```python
from build123d import *

# Parameters (mm, degrees)
F1_DEPTH = 25.4
F2_DEPTH = 50.8


with BuildPart() as f1:
    # F0 (on Top) → F1 (new body)
    with BuildSketch(Plane.XY):
        with BuildLine():
            Line((-22.589232, -50.8), (0, -50.8))
            Line((0, -50.8), (22.589232, -50.8))
            ThreePointArc((22.589232, -50.8), (29.879351, -49.349905), (36.059616, -45.220384))
            Line((36.059616, -45.220384), (45.220384, -36.059616))
            ThreePointArc((45.220384, -36.059616), (49.349905, -29.879351), (50.8, -22.589232))
            Line((50.8, -22.589232), (50.8, 0))
            Line((50.8, 0), (50.8, 22.589232))
            ThreePointArc((50.8, 22.589232), (49.349905, 29.879351), (45.220384, 36.059616))
            Line((45.220384, 36.059616), (36.059616, 45.220384))
            ThreePointArc((36.059616, 45.220384), (29.879351, 49.349905), (22.589232, 50.8))
            Line((22.589232, 50.8), (0, 50.8))
            Line((0, 50.8), (-22.589232, 50.8))
            ThreePointArc((-22.589232, 50.8), (-29.879351, 49.349905), (-36.059616, 45.220384))
            Line((-36.059616, 45.220384), (-45.220384, 36.059616))
            ThreePointArc((-45.220384, 36.059616), (-49.349905, 29.879351), (-50.8, 22.589232))
            Line((-50.8, 22.589232), (-50.8, 0))
            Line((-50.8, 0), (-50.8, -22.589232))
            ThreePointArc((-50.8, -22.589232), (-49.349905, -29.879351), (-45.220384, -36.059616))
            Line((-45.220384, -36.059616), (-36.059616, -45.220384))
            ThreePointArc((-36.059616, -45.220384), (-29.879351, -49.349905), (-22.589232, -50.8))
        make_face()
    extrude(amount=F1_DEPTH)

    # F0 (on Top) → F2 (join)
    with BuildSketch(Plane.XY):
        with BuildLine():
            ThreePointArc((54.20064, -45.039872), (61.083175, -34.739431), (63.5, -22.589232))
            Line((63.5, -22.589232), (63.5, 0))
            Line((63.5, 0), (63.5, 22.589232))
            ThreePointArc((63.5, 22.589232), (61.083175, 34.739431), (54.20064, 45.039872))
            Line((54.20064, 45.039872), (45.039872, 54.20064))
            ThreePointArc((45.039872, 54.20064), (34.739431, 61.083175), (22.589232, 63.5))
            Line((22.589232, 63.5), (0, 63.5))
            Line((0, 63.5), (-22.589232, 63.5))
            ThreePointArc((-22.589232, 63.5), (-34.739431, 61.083175), (-45.039872, 54.20064))
            Line((-45.039872, 54.20064), (-54.20064, 45.039872))
            ThreePointArc((-54.20064, 45.039872), (-61.083175, 34.739431), (-63.5, 22.589232))
            Line((-63.5, 22.589232), (-63.5, 0))
            Line((-63.5, 0), (-63.5, -22.589232))
            ThreePointArc((-63.5, -22.589232), (-61.083175, -34.739431), (-54.20064, -45.039872))
            Line((-54.20064, -45.039872), (-45.039872, -54.20064))
            ThreePointArc((-45.039872, -54.20064), (-34.739431, -61.083175), (-22.589232, -63.5))
            Line((-22.589232, -63.5), (0, -63.5))
            Line((0, -63.5), (22.589232, -63.5))
            ThreePointArc((22.589232, -63.5), (34.739431, -61.083175), (45.039872, -54.20064))
            Line((45.039872, -54.20064), (54.20064, -45.039872))
        make_face()
        with BuildLine():
            Line((22.589232, -50.8), (0, -50.8))
            Line((0, -50.8), (-22.589232, -50.8))
            ThreePointArc((-22.589232, -50.8), (-29.879351, -49.349905), (-36.059616, -45.220384))
            Line((-36.059616, -45.220384), (-45.220384, -36.059616))
            ThreePointArc((-45.220384, -36.059616), (-49.349905, -29.879351), (-50.8, -22.589232))
            Line((-50.8, -22.589232), (-50.8, 0))
            Line((-50.8, 0), (-50.8, 22.589232))
            ThreePointArc((-50.8, 22.589232), (-49.349905, 29.879351), (-45.220384, 36.059616))
            Line((-45.220384, 36.059616), (-36.059616, 45.220384))
            ThreePointArc((-36.059616, 45.220384), (-29.879351, 49.349905), (-22.589232, 50.8))
            Line((-22.589232, 50.8), (0, 50.8))
            Line((0, 50.8), (22.589232, 50.8))
            ThreePointArc((22.589232, 50.8), (29.879351, 49.349905), (36.059616, 45.220384))
            Line((36.059616, 45.220384), (45.220384, 36.059616))
            ThreePointArc((45.220384, 36.059616), (49.349905, 29.879351), (50.8, 22.589232))
            Line((50.8, 22.589232), (50.8, 0))
            Line((50.8, 0), (50.8, -22.589232))
            ThreePointArc((50.8, -22.589232), (49.349905, -29.879351), (45.220384, -36.059616))
            Line((45.220384, -36.059616), (36.059616, -45.220384))
            ThreePointArc((36.059616, -45.220384), (29.879351, -49.349905), (22.589232, -50.8))
        make_face(mode=Mode.SUBTRACT)
    extrude(amount=F2_DEPTH)


solid = f1.part
```
The listing builds one solid part. Answer for the finished solid, in the listing's coordinates (mm). A direction names the side the tool comes from. Coordinates: 2 decimals unless noted, no trailing zeros. Write each loop counter-clockwise with the first axis right and the second up, starting at its lowest first coordinate (ties: lowest second). Pieces come first, ordered by that corner, then holes. Notation, with made-up numbers: (56, 31.5) - (100, 31.5) arc R20 cw to (100, 59.5) - close; hole circle Ø6 at (-38.5, 36.25). An arc over 180 degrees is marked (long way). Return JSON: item names as keys, results as strings. Group by question number.
Q1. For a pull along X with two mould halves and no side action, classify faces 1 (the cylindrical face through (-61.016, 34.901, 25.044)), 2 (the cylindrical face through (-49.39, 29.78, 37.92)), 3 (the flat face through (-1, 1, 0)) as +X half, -X half, draft (parallel to the pull), parting line (faces both ways), or undercut.
Q2. Flat-ended cylindrical pins translate along their axes: pin 1 Ø5 at (x, z) = (-42, 15) entering from -Y; pin 2 Ø5 at (x, y) = (37, -5.5) entering from -Z; pin 3 Ø6 at (x, y) = (-28.5, -2.5) entering from +Z; pin 4 Ø6 at (y, z) = (28.5, 45.5) entering from -X. Find the tip coordinate at first contact, or state that the pin passes through.
Q3. Which of the six approach directions +Z, -Z, +X, -X, +Y, -Y give full straight-line access (tool end or side, diameter ignored) to faces 4 (the cylindrical face through (34.901, 61.016, 25.044)), 5 (the flat face through (50.8, 0, 38))?
Q4. Find the intervals of material crossed by line 1 along X through (y, z) = (-20.5, 31.5); line 2 along Z through (x, y) = (31, 36), in increasing order. Write a range as [from, to].
Q5. The part is cut by section D-D on z = 22.5. Write down the section's boundary in (x, y), and give its area (3 significant figures).
Q6. The part is cut by section A-A on x = -10. Write down the section's boundary in (y, z).
Evaluation:
{
 "1": {"face 1": "-X half", "face 2": "undercut", "face 3": "draft"},
 "2": {"pin 1": "stops at y = -58.62", "pin 2": "stops at z = 0", "pin 3": "stops at z = 25.4", "pin 4": "stops at x = -63.37"},
 "3": {"face 4": "+Z, -Z, +X, +Y", "face 5": "+Z"},
 "4": {"line 1": "x = [-63.5, -50.8], [50.8, 63.5]", "line 2": "z = [0, 25.4]"},
 "5": {"outline": "(-63.5, -22.59) arc R31.75 ccw to (-54.2, -45.04) - (-45.04, -54.2) arc R31.75 ccw to (-22.59, -63.5) - (22.59, -63.5) arc R31.75 ccw to (45.04, -54.2) - (54.2, -45.04) arc R31.75 ccw to (63.5, -22.59) - (63.5, 22.59) arc R31.75 ccw to (54.2, 45.04) - (45.04, 54.2) arc R31.75 ccw to (22.59, 63.5) - (-22.59, 63.5) arc R31.75 ccw to (-45.04, 54.2) - (-54.2, 45.04) arc R31.75 ccw to (-63.5, 22.59) - close", "area": "14,400 mm2"},
 "6": {"outline": "(-63.5, 0) - (63.5, 0) - (63.5, 50.8) - (50.8, 50.8) - (50.8, 25.4) - (-50.8, 25.4) - (-50.8, 50.8) - (-63.5, 50.8) - close"}
}
